```python
from build123d import *

# Parameters (mm, degrees)
SKETCH1_W           = 12.8524
SKETCH1_H           = 23.8252
BOSS_EXTRUDE1_DEPTH = 13.97
SKETCH2_R           = 5.953125
BOSS_EXTRUDE2_DEPTH = 7.540625
SKETCH3_W           = 1.5875
SKETCH3_H           = 0.79375
CUT_EXTRUDE1_DEPTH  = 5.953125
SKETCH4_R           = 1.790559095
BOSS_EXTRUDE3_DEPTH = 10.5918


with BuildPart() as part:
    # Sketch1 → Boss-Extrude1 (new body)
    with BuildSketch(Plane(origin=(0, 0, 0), x_dir=(1, 0, 0), z_dir=(0, 1, 0))):
        with Locations((-8.41333272, -1.665416216)):
            Rectangle(SKETCH1_W, SKETCH1_H)
    extrude(amount=BOSS_EXTRUDE1_DEPTH)

    # Sketch2 → Boss-Extrude2 (add)
    with BuildSketch(Plane(origin=(0, 13.97, 0), x_dir=(1, 0, 0), z_dir=(0, 1, 0))):
        with Locations((-8.41333272, -1.665416216)):
            Circle(SKETCH2_R)
    extrude(amount=BOSS_EXTRUDE2_DEPTH)

    # Sketch3 → Cut-Extrude1 (cut)
    with BuildSketch(Plane(origin=(0, 21.510625, 0), x_dir=(1, 0, 0), z_dir=(0, 1, 0))):
        with Locations((-8.41333272, -7.221666216)):
            Rectangle(SKETCH3_W, SKETCH3_H)
    extrude(amount=-CUT_EXTRUDE1_DEPTH, mode=Mode.SUBTRACT)

    # Sketch4 → Boss-Extrude3 (add)
    with BuildSketch(Plane(origin=(0, 21.510625, 0), x_dir=(1, 0, 0), z_dir=(0, 1, 0))):
        with Locations((-8.41333272, -1.665416216)):
            Circle(SKETCH4_R)
    extrude(amount=BOSS_EXTRUDE3_DEPTH)


solid = part.part
```
Here's how the part is built. I have some questions about the finished solid (model axes, mm). A direction names the side the tool comes from. Coordinates: 2 decimals unless noted, no trailing zeros. Write each loop counter-clockwise with the first axis right and the second up, starting at its lowest first coordinate (ties: lowest second). Pieces come first, ordered by that corner, then holes. Notation, with made-up numbers: (55, 2) -> (62, 2) arc R20 ccw to (62, 26) -> close; hole circle Ø2 at (-14.75, 84.25). An arc over 180 degrees is marked (long way). Use a Markdown table: item, result. Add a question column.
(1) Please list where these lines run through material, in increasing order: line 1 (Y direction, x = -8, z = 9.75); line 2 (X direction, y = 20.5, z = 7); line 3 (Y direction, x = -11.25, z = -1).
(2) We'd pull the mould along X, two halves only. Please class faces 3 (the flat face through (-11, 13.97, -4)), 4 (the cylindrical face through (-14.36, 17.69, 1.4)), 5 (the flat face through (-8, 19, 6.825)), 6 (the flat face through (-1.987, 7, 2)): +X half, -X half, draft (parallel to the pull), parting line (faces both ways), or undercut.
(3) If we section it at A-A, the plane z = 1: Write out the boundary of the cut face in (x, y).
(4) If we section it at B-B, the plane y = 20: Write out the boundary of the cut face in (x, z), and give its area (3 significant figures).
(5) If we section it at D-D, the plane y = 15: Write out the boundary of the cut face in (x, z), and give its area (3 significant figures).
(6) I'm going to push flat-ended pins straight in: P1, Ø4, axis at x = -10, z = -2.5, coming from the +Y side; P2, Ø1.3, axis at x = -8.5, y = 17, coming from the +Z side; P3, Ø1, axis at x = -13, y = 18, coming from the -Z side; P4, Ø3, axis at x = -8.5, z = 3.5, coming from the -Y side. Where does each tip first touch, or does it pass through?
(7) For faces 1 (the flat face through (-9, 0, 1)), 2 (the flat face through (-10, 21.511, 3)), which set-ups out of +Z, -Z, +X, -X, +Y, -Y let a thin tool reach every point of the face, with its end or its side?
(8) If we section it at C-C, the plane z = -3.5: Write out the boundary of the cut face in (x, y), and give its area (3 significant figures).
Outcome:
| question | item | result |
|---|---|---|
| 1 | line 1 | y = 0 to 13.97 |
| 1 | line 2 | x = -11.06 to -9.21, -7.62 to -5.77 |
| 1 | line 3 | y = 0 to 21.51 |
| 2 | face 3 | draft |
| 2 | face 4 | parting line |
| 2 | face 5 | undercut |
| 2 | face 6 | +X half |
| 3 | outline | (-14.84, 0) -> (-1.99, 0) -> (-1.99, 13.97) -> (-2.5, 13.97) -> (-2.5, 21.51) -> (-6.75, 21.51) -> (-6.75, 32.1) -> (-10.08, 32.1) -> (-10.08, 21.51) -> (-14.33, 21.51) -> (-14.33, 13.97) -> (-14.84, 13.97) -> close |
| 4 | outline | (-9.21, 6.82) -> (-9.21, 7.57) arc R5.95 ccw (long way) to (-7.62, 7.57) -> (-7.62, 6.82) -> close |
| 4 | area | 110 mm^2 |
| 5 | outline | circle Ø11.91 at (-8.41, 1.67) |
| 5 | area | 111 mm^2 |
| 6 | P1 | stops at y = 21.51 |
| 6 | P2 | stops at z = 6.82 |
| 6 | P3 | stops at z = -2.66 |
| 6 | P4 | stops at y = 0 |
| 7 | face 1 | +Z, -Z, +X, -X, -Y |
| 7 | face 2 | +Y |
| 8 | outline | (-14.84, 0) -> (-1.99, 0) -> (-1.99, 13.97) -> (-5.45, 13.97) -> (-5.45, 21.51) -> (-11.37, 21.51) -> (-11.37, 13.97) -> (-14.84, 13.97) -> close |
| 8 | area | 224 mm^2 |
